Can you work these out from the model? Positions are in its coordinate system, mm. Face numbers are marked on the shaded views. A direction names the side the tool comes from. Round coordinates to 2 decimals unless told otherwise and drop trailing zeros. Order: outer loops, then holes, each group sorted by start corner. A loop starts at its lowest first (then second) coordinate and runs counter-clockwise, first axis right, second up. Notation, with made-up numbers: M 88.25,52 L 112.25,52 A23 ccw 112.25,62 Z; hole C 41.5,23 d3. An arc over 180 degrees is marked long. Answer as a JSON object with one key per item and string values. Group by question number.
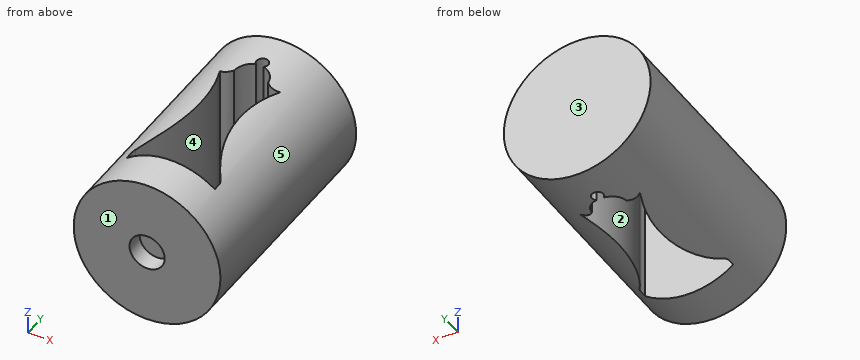
from build123d import *

# Parameters (mm, degrees)
SKETCH2_R               = 12.5
BOSS_EXTRUDE1_DEPTH     = 20
CUT_EXTRUDE1_DEPTH      = 13.5
CUT_EXTRUDE1_DEPTH_BACK = 13.5
SKETCH4_R               = 3
CUT_EXTRUDE2_DEPTH      = 3


with BuildPart() as part:
    # Sketch2 → Boss-Extrude1 (new body, symmetric)
    with BuildSketch(Plane(origin=(0, 0, 0), x_dir=(1, 0, 0), z_dir=(0, 1, 0))):
        Circle(SKETCH2_R)
    extrude(amount=BOSS_EXTRUDE1_DEPTH, both=True)

    # Sketch3 → Cut-Extrude1 (cut, two sides)
    with BuildSketch(Plane.XY) as cut_extrude1_sk:
        with BuildLine():
            Line((-7.5, -13), (7.5, -13))
            Line((7.5, -13), (7.5, -11.75))
            ThreePointArc((7.5, -11.75), (7.429735441, -11.282497399), (7.225150448, -10.856304049))
            ThreePointArc((7.225150448, -10.856304049), (3.577993471, -1.282835033), (4.615823257, 8.909121225))
            Line((4.615823257, 8.909121225), (5.118882067, 10.357861534))
            ThreePointArc((5.118882067, 10.357861534), (3.945658152, 10.08267593), (2.899801007, 10.681311299))
            ThreePointArc((2.899801007, 10.681311299), (2.188817627, 12.324233844), (0.651338796, 13.241212959))
            ThreePointArc((0.651338796, 13.241212959), (0, 15), (-0.651338796, 13.241212959))
            ThreePointArc((-0.651338796, 13.241212959), (-2.188817627, 12.324233844), (-2.899801007, 10.681311299))
            ThreePointArc((-2.899801007, 10.681311299), (-3.945658152, 10.08267593), (-5.118882067, 10.357861534))
            Line((-5.118882067, 10.357861534), (-4.615823257, 8.909121225))
            ThreePointArc((-4.615823257, 8.909121225), (-3.577993471, -1.282835033), (-7.225150448, -10.856304049))
            ThreePointArc((-7.225150448, -10.856304049), (-7.429735441, -11.282497399), (-7.5, -11.75))
            Line((-7.5, -11.75), (-7.5, -13))
        make_face()
    extrude(amount=CUT_EXTRUDE1_DEPTH, mode=Mode.SUBTRACT)
    extrude(cut_extrude1_sk.sketch, amount=-CUT_EXTRUDE1_DEPTH_BACK, mode=Mode.SUBTRACT)

    # Sketch4 → Cut-Extrude2 (cut)
    with BuildSketch(Plane(origin=(0, -20, 0), x_dir=(-1, 0, 0), z_dir=(0, -1, 0))):
        Circle(SKETCH4_R)
    extrude(amount=-CUT_EXTRUDE2_DEPTH, mode=Mode.SUBTRACT)


solid = part.part
Item 1: If we mould it in two halves opening along Y, with no side actions, what happens to the marked faces 1, 2 and 3? For each: +Y half, -Y half, draft (parallel to the pull), parting line (faces both ways), or undercut.
Item 2: Suppose I cut it at B-B, the plane z = 0. Write out the boundary of the cut face in (x, y), and give its area (3 significant figures).
Item 3: Suppose I cut it at D-D, the plane z = 10.75. Write out the boundary of the cut face in (x, y).
Item 4: I'm going to push flat-ended pins straight in: pin 1 Ø8 at (x, z) = (0, 0) entering from -Y; pin 2 Ø3 at (y, z) = (-1, -9.5) entering from -X; pin 3 Ø8 at (x, y) = (2.5, -3) entering from -Z; pin 4 Ø8 at (x, y) = (5.5, 5.5) entering from +Z. Where does each tip first touch, or does it pass through?
Item 5: Suppose I cut it at C-C, the plane y = 5. Write out the boundary of the cut face in (x, z), and give its area (3 significant figures).
Item 6: I need wall thicknesses on line 1 (Z direction, x = 0, y = -19.1); line 2 (Y direction, x = 0, z = 6.5). Which ranges of each line are inside material? Lowest first, please.
Item 7: On a 3-axis mill with a long thin cutter (end or side, diameter ignored), from which of +Z, -Z, +X, -X, +Y, -Y can I reach the whole of each face in a straight line? I mean the marked faces 4 and 5. Say none if no direction works.
Item 8: Suppose I cut it at A-A, the plane x = 0. Write out the boundary of the cut face in (y, z), and give its area (3 significant figures).
Computed:
{
 "1": {"face 1": "-Y half", "face 2": "undercut", "face 3": "+Y half"},
 "2": {"outline": "M -12.5,-20 L -3,-20 L -3,-17 L 3,-17 L 3,-20 L 12.5,-20 L 12.5,20 L -12.5,20 Z; hole M -7.5,-13 L 7.5,-13 L 7.5,-11.75 A1.59 ccw 7.23,-10.86 A22.21 cw 4.62,8.91 L 5.12,10.36 A1.64 cw 2.9,10.68 A2.91 ccw 0.65,13.24 A1 ccw long -0.65,13.24 A2.91 ccw -2.9,10.68 A1.64 cw -5.12,10.36 L -4.62,8.91 A22.21 cw -7.23,-10.86 A1.59 ccw -7.5,-11.75 Z", "area": "750 mm^2"},
 "3": {"outline": "M -6.38,-20 L 6.38,-20 L 6.38,-13 L -6.38,-13 Z; M -6.38,-9.51 A22.21 ccw -4.62,8.91 L -5.12,10.36 A1.64 ccw -2.9,10.68 A2.91 cw -0.65,13.24 A1 cw long 0.65,13.24 A2.91 cw 2.9,10.68 A1.64 ccw 5.12,10.36 L 4.62,8.91 A22.21 ccw 6.38,-9.51 L 6.38,20 L -6.38,20 Z"},
 "4": {"pin 1": "stops at y = -20", "pin 2": "stops at x = -9.6", "pin 3": "stops at z = -12.03", "pin 4": "stops at z = 12.03"},
 "5": {"outline": "M -3.65,-11.96 L -3.65,11.96 A12.5 ccw Z; M 3.65,-11.96 A12.5 ccw 3.65,11.96 Z", "area": "311 mm^2"},
 "6": {"line 1": "z = -12.5 to -3, 3 to 12.5", "line 2": "y = -20 to -13, 15 to 20"},
 "7": {"face 4": "+Z, -Z", "face 5": "+Y, -Y"},
 "8": {"outline": "M -20,-12.5 L -13,-12.5 L -13,12.5 L -20,12.5 L -20,3 L -17,3 L -17,-3 L -20,-3 Z; M 15,-12.5 L 20,-12.5 L 20,12.5 L 15,12.5 Z", "area": "282 mm^2"}
}
